Autodesk Inventor part; units mm, degrees
ref_plane "YZ Plane" through (0, 0, 0) normal (1, 0, 0) x (0, 1, 0)
ref_plane "XZ Plane" through (0, 0, 0) normal (0, 1, 0) x (-1, 0, 0)
ref_plane "XY Plane" through (0, 0, 0) normal (0, 0, 1) x (1, 0, 0)
sketch "Sketch1" plane through (0, 0, 0) normal (0, 0, 1) x (1, 0, 0)
  circle A0 centre (0, 0) radius 3.75
  circle A1 centre (0, 0) radius 15
  arc A2 (-0.5916, -14.9883) -> (-0.5916, -14.9883) centre (0, 0) ccw
  circle A3 centre (0, 38.847) radius 6
  circle A4 centre (0, 0) radius 11
  line L0 (5.8417, 40.216) -> (14.0107, 5.3571)
  line L1 (-14.0107, 5.3571) -> (-5.8417, 40.216)
  point P0 (-13.5955, 6.3373)
  point P1 (13.5955, 6.3373)
  point P2 (23.3721, 30.2282)
  dimension "d0" = 30
  dimension "d3" = 12
  dimension "d8" = 22
  dimension "d10" = 38.847
extrude "Extrusion1" add sketch "Sketch1" along normal blind 9 contours A1 | A1 L1 A3 L0 | A3
sketch "Sketch2" plane through (0, 0, 9) normal (0, 0, 1) x (1, 0, 0)
  circle A0 centre (0, 38.847) radius 6
  arc A1 (5.8417, 40.216) -> (-5.8417, 40.216) centre (0, 38.847) ccw
  circle A2 centre (0, 38.847) radius 1.4
  point P0 (0, 0)
  dimension "d4" = 12
  dimension "d11" = 2.8
extrude "Extrusion2" add sketch "Sketch2" along normal blind 6
sketch "Sketch3" plane through (0, 0, 0) normal (0, 0, -1) x (-1, 0, 0)
  arc A0 (5.8417, 40.216) -> (-5.8417, 40.216) centre (0, 38.847) ccw
  circle A1 centre (0, 38.847) radius 6
  point P0 (0, 0)
  dimension "d12" = 12
extrude "Extrusion3" cut sketch "Sketch3" against normal blind 8
properties part number "ClickSpringBacking"
Can you work these out from the model? Positions are in its coordinate system, mm. A direction names the side the tool comes from. Round coordinates to 2 decimals unless told otherwise and drop trailing zeros. Loops run counter-clockwise (first coordinate to the right, second up) from the corner with the lowest first, then second, coordinate; pieces in that order, holes last.
Item 1: If we mould it in two halves opening along X, with no side actions, what happens to faces 1 (the cylindrical face through (-2.38, 10.74, 4.44)), 2 (the flat face through (9.87, 23.03, 4.44)), 3 (the flat face through (-9.983, 22.543, 4.437)), 4 (the flat face through (1.2, 37.6, 15))? For each: +X half, -X half, draft (parallel to the pull), parting line (faces both ways), or undercut.
Item 2: Suppose I cut it at B-B, the plane y = 0. Write out the boundary of the cut face in (x, z), then the cut area to 3 significant figures.
Item 3: Suppose I cut it at D-D, the plane y = 7. Write out the boundary of the cut face in (x, z).
Item 4: Will these pins go through, and if not, where does the flat tip stop? pin 1 Ø5 at (x, z) = (-0.5, 12.5) entering from -Y; pin 2 Ø2 at (x, z) = (6, 2.5) entering from -Y; pin 3 Ø3.5 at (x, y) = (0, 38.847) entering from -Z.
Item 5: Which directions (+Z, -Z, +X, -X, +Y, -Y) give clear straight access to the entire face, cutting with the end or side of a thin tool? Please do faces 5 (the cylindrical face through (-0.113, 44.846, 11.958)), 6 (the cylindrical face through (0.15, 32.85, 3.94)), 7 (the flat face through (0, 39, 9)).
Item 6: Suppose I cut it at C-C, the plane z = 4. Write out the boundary of the cut face in (x, y), then the cut area to 3 significant figures.
Item 7: Please list where these lines run through material, in increasing order: L1, parallel to Y at x = 0, z = 11.5; L2, parallel to Z at x = -11.5, y = 1; L3, parallel to Y at x = 0, z = 2.5.
Item 8: Suppose I cut it at A-A, the plane x = 0. Write out the boundary of the cut face in (y, z).
Reported:
1. face 1: undercut
1. face 2: +X half
1. face 3: -X half
1. face 4: draft
2. outline: (-15, 0) - (-11, 0) - (-11, 9) - (-15, 9) - close; (11, 0) - (15, 0) - (15, 9) - (11, 9) - close
2. area: 72.0 mm2
3. outline: (-13.63, 0) - (-8.49, 0) - (-8.49, 9) - (-13.63, 9) - close; (8.49, 0) - (13.63, 0) - (13.63, 9) - (8.49, 9) - close
4. pin 1: stops at y = 32.85
4. pin 2: stops at y = -14.14
4. pin 3: stops at z = 8
5. face 5: +Z, -Z, +Y
5. face 6: -Z
5. face 7: +Z
6. outline: (-14.01, 5.36) arc R15 ccw (long way) to (14.01, 5.36) - (5.85, 40.2) arc R6 cw (long way) to (-5.85, 40.2) - close; hole circle Ø22 at (0, 0)
6. area: 750 mm2
7. L1: y = 32.85 to 37.45, 40.25 to 44.85
7. L2: z = 0 to 9
7. L3: y = -15 to -11, 11 to 32.85
8. outline: (-15, 0) - (-11, 0) - (-11, 9) - (-15, 9) - close; (11, 0) - (32.85, 0) - (32.85, 8) - (44.85, 8) - (44.85, 15) - (40.25, 15) - (40.25, 9) - (37.45, 9) - (37.45, 15) - (32.85, 15) - (32.85, 9) - (11, 9) - close
